from build123d import *

# Parameters (mm, degrees)
BOSS_EXTRUDE1_DEPTH      = 1.27
REVOLVE3_ANGLE           = 90
SKETCH6_W                = 4.862612613
SKETCH6_H                = 1.27
BOSS_EXTRUDE3_DEPTH      = 7.935530078
BOSS_EXTRUDE4_DEPTH      = 3.81
BOSS_EXTRUDE4_DEPTH_BACK = 6.35
SKETCH10_W               = 4.862612613
SKETCH10_H               = 7.935530078
FILLET7_R                = 5.08
FILLET10_R               = 5.08
SKETCH13_R               = 1.651
CUT_EXTRUDE2_DEPTH       = 55.372
SKETCH14_W               = 2.286
SKETCH14_H               = 11.368095807
CUT_EXTRUDE3_DEPTH       = 55.372
FILLET15_RADIUS          = 3.967765039
FILLET15_LENGTH          = 2.576612613
FILLET16_RADIUS          = 3.967765039
FILLET16_LENGTH          = 2.576612613
CUT_EXTRUDE4_DEPTH       = 55.372
CUT_EXTRUDE7_DEPTH       = 55.88
SKETCH19_W               = 2.576612613
SKETCH19_H               = 3.428576371
BOSS_EXTRUDE5_DEPTH      = 3.81
FILLET17_R               = 3.302
FILLET18_R               = 3.302


with BuildPart() as part:
    # Sketch1 → Boss-Extrude1 (new body)
    with BuildSketch(Plane(origin=(0, 0, 0), x_dir=(1, 0, 0), z_dir=(0, 1, 0))):
        with BuildLine():
            Line((-18.44626818, 0), (-13.583655567, 0))
            ThreePointArc((-13.583655567, 0), (5.056359448, 18.640015015), (23.696374463, 0))
            Line((23.696374463, 0), (28.558987076, 0))
            ThreePointArc((28.558987076, 0), (5.056359448, 23.502627628), (-18.44626818, 0))
        make_face()
    extrude(amount=BOSS_EXTRUDE1_DEPTH)

    # Sketch4 → Revolve3 (revolve)
    with BuildSketch(Plane(origin=(0, 1.27, 0), x_dir=(1, 0, 0), z_dir=(0, 1, 0))):
        with BuildLine():
            Line((23.696374463, 0), (28.014374463, 0))
            ThreePointArc((28.014374463, 0), (5.056359448, 22.958015015), (-17.901655567, 0))
            Line((-17.901655567, 0), (-13.583655567, 0))
            ThreePointArc((-13.583655567, 0), (5.056359448, 18.640015015), (23.696374463, 0))
        make_face()
    revolve(axis=Axis((-17.901655567, 1.27, 0), (1, 0, 0)), revolution_arc=REVOLVE3_ANGLE)

    # Sketch6 → Boss-Extrude3 (add)
    with BuildSketch(Plane.XY):
        with Locations((-16.014961873, 0.635)):
            Rectangle(SKETCH6_W, SKETCH6_H)
        with Locations((26.12768077, 0.635)):
            Rectangle(SKETCH6_W, SKETCH6_H)
    extrude(amount=BOSS_EXTRUDE3_DEPTH)

    # Sketch10 → Boss-Extrude4 (add, two sides: drawn at the far end of the back side and taken through both)
    with BuildSketch(Plane(origin=(0, 1.27, 0), x_dir=(1, 0, 0), z_dir=(0, 1, 0)).offset(-BOSS_EXTRUDE4_DEPTH_BACK)):
        with Locations((-16.014961873, -3.967765039)):
            Rectangle(SKETCH10_W, SKETCH10_H)
        with Locations((26.12768077, -3.967765039)):
            Rectangle(SKETCH10_W, SKETCH10_H)
    extrude(amount=BOSS_EXTRUDE4_DEPTH + BOSS_EXTRUDE4_DEPTH_BACK)

    # Fillet7
    fillet7_edges = [part.edges().sort_by_distance(p)[0] for p in [
        (-16.014961873, 5.08, 7.935530078),
    ]]
    fillet(fillet7_edges, radius=FILLET7_R)

    # Fillet10
    fillet10_edges = [part.edges().sort_by_distance(p)[0] for p in [
        (26.127680769, 5.08, 7.935530078),
    ]]
    fillet(fillet10_edges, radius=FILLET10_R)

    # Sketch13 → Cut-Extrude2 (cut)
    with BuildSketch(Plane.ZY.offset(18.44626818)):
        with Locations((3.428576371, 0)):
            Circle(SKETCH13_R)
    extrude(amount=-CUT_EXTRUDE2_DEPTH, mode=Mode.SUBTRACT)

    # Sketch14 → Cut-Extrude3 (cut)
    with BuildSketch(Plane(origin=(0, 5.08, 0), x_dir=(1, 0, 0), z_dir=(0, 1, 0))):
        with Locations((27.415987076, -5.684047904)):
            Rectangle(SKETCH14_W, SKETCH14_H)
        with Locations((-17.30326818, -5.684047904)):
            Rectangle(SKETCH14_W, SKETCH14_H)
    extrude(amount=-CUT_EXTRUDE3_DEPTH, mode=Mode.SUBTRACT)

    # Fillet15: full round fillet: the end face becomes a half cylinder, R = half its width
    fillet15_face = Plane((24.984680769, -5.08, 3.967765039), x_dir=(1, 0, 0), z_dir=(0, -1, 0))  # on the end face: x along it, z out of the body
    fillet15_slab = fillet15_face.offset(-FILLET15_RADIUS / 2) * Box(FILLET15_LENGTH, 2 * FILLET15_RADIUS, FILLET15_RADIUS, mode=Mode.PRIVATE)  # the body's end, R deep
    fillet15_round = Plane((24.984680769, -1.112234961, 3.967765039), x_dir=(0, -1, 0), z_dir=(1, 0, 0)) * Cylinder(FILLET15_RADIUS, FILLET15_LENGTH, mode=Mode.PRIVATE)  # its axis R under the face
    add(fillet15_slab - fillet15_round, mode=Mode.SUBTRACT)

    # Fillet16: full round fillet: the end face becomes a half cylinder, R = half its width
    fillet16_face = Plane((-14.871961873, -5.08, 3.967765039), x_dir=(-1, 0, 0), z_dir=(0, -1, 0))  # on the end face: x along it, z out of the body
    fillet16_slab = fillet16_face.offset(-FILLET16_RADIUS / 2) * Box(FILLET16_LENGTH, 2 * FILLET16_RADIUS, FILLET16_RADIUS, mode=Mode.PRIVATE)  # the body's end, R deep
    fillet16_round = Plane((-14.871961873, -1.112234961, 3.967765039), x_dir=(0, -1, 0), z_dir=(-1, 0, 0)) * Cylinder(FILLET16_RADIUS, FILLET16_LENGTH, mode=Mode.PRIVATE)  # its axis R under the face
    add(fillet16_slab - fillet16_round, mode=Mode.SUBTRACT)

    # Sketch16 → Cut-Extrude4 (cut)
    with BuildSketch(Plane(origin=(26.272987076, 0, 0), x_dir=(0, 0, -1), z_dir=(1, 0, 0))):
        with BuildLine():
            ThreePointArc((0, 0), (-3.716578938, -3.862364093), (-7.935530078, -0.55611748))
            ThreePointArc((-7.935530078, -0.55611748), (-3.630565744, -5.089731167), (0, 0))
        make_face()
    extrude(amount=-CUT_EXTRUDE4_DEPTH, mode=Mode.SUBTRACT)

    # Sketch18 → Cut-Extrude7 (cut)
    with BuildSketch(Plane(origin=(26.272987076, 0, 0), x_dir=(0, 0, -1), z_dir=(1, 0, 0))):
        with BuildLine():
            Line((-3.428576371, 3.428576371), (0, 3.428576371))
            Line((0, 3.428576371), (0, 5.467356317))
            Line((0, 5.467356317), (-9.031573881, 5.467356317))
            Line((-9.031573881, 5.467356317), (-9.031573881, -4.486785293))
            Line((-9.031573881, -4.486785293), (0, -4.486785293))
            Line((0, -4.486785293), (0, 0))
            ThreePointArc((0, 0), (-5.852945973, -2.424369602), (-3.428576371, 3.428576371))
        make_face()
    extrude(amount=-CUT_EXTRUDE7_DEPTH, mode=Mode.SUBTRACT)

    # Sketch19 → Boss-Extrude5 (add)
    with BuildSketch(Plane(origin=(0, 3.428576371, 0), x_dir=(1, 0, 0), z_dir=(0, 1, 0))):
        with Locations((24.98468077, -1.714288186)):
            Rectangle(SKETCH19_W, SKETCH19_H)
        with Locations((-14.871961874, -1.714288186)):
            Rectangle(SKETCH19_W, SKETCH19_H)
    extrude(amount=BOSS_EXTRUDE5_DEPTH)

    # Fillet17
    fillet17_edges = [part.edges().sort_by_distance(p)[0] for p in [
        (24.984680769, 7.238576371, 3.428576371),
    ]]
    fillet(fillet17_edges, radius=FILLET17_R)

    # Fillet18
    fillet18_edges = [part.edges().sort_by_distance(p)[0] for p in [
        (-14.871961873, 7.238576371, 3.428576371),
    ]]
    fillet(fillet18_edges, radius=FILLET18_R)


solid = part.part
CAD build for the part. Positions are in the model's coordinates, mm. A direction names the side the tool comes from. Give positions to 0.01 mm unless a question says otherwise; leave off trailing zeros. Loops run counter-clockwise (first coordinate to the right, second up) from the corner with the lowest first, then second, coordinate; pieces in that order, holes last. Notation, with made-up numbers: M 26,88.5 L 38,88.5 A34 cw 38,119.5 Z; hole C 35.5,34.5 d5. An arc over 180 degrees is marked long. Write each question's results on one line, items separated by ' | '.
Q1. Probe probe 1 along X at (y, z) = (5.5, 3); probe 2 along X at (y, z) = (1, -10); probe 3 along Z at (x, y) = (26, 0.5). List the from-to ranges inside material, lowest first.
Geometry check:
probe 1: x = -16.16 to -13.58, 23.7 to 26.27 | probe 2: x = -16.21 to -10.67, 20.79 to 26.33 | probe 3: z = -10.66 to 1.86, 5 to 6.82
Q2. Which spindle directions (+Z, -Z, +X, -X, +Y, -Y) get a long thin tool onto all of the face, cutting with end or side? Do faces 1 (the face through (7, 0, -19)), 2 (the face through (4.95, 1.27, -23.12)), 3 (the face through (4.646, 0.626, -18.636)), 4 (the face through (23.696, 2, 3)), 5 (the face through (26.273, 2, 3)). Say none if no direction does.
Geometry check:
face 1: -Z, +X, -X, -Y | face 2: -Z, +Y | face 3: +Z, -Y | face 4: +Z, +Y, -Y | face 5: +Z, +X, +Y, -Y
Q3. Band-saw the part on D-D on y = 4.75. Write the cut outline in (x, z).
Geometry check:
outline: M -17.64,0 A22.69 ccw 27.75,0 L 26.27,0 L 26.27,3.33 L 23.7,3.33 L 23.7,0 L 23.37,0 A18.31 cw -13.26,0 L -13.58,0 L -13.58,3.33 L -16.16,3.33 L -16.16,0 Z
Q4. Mould opens along Z. For faces 6 (the face through (24.97, 0.07, 1.78)), 7 (the face through (-14.89, 0.07, 1.78)), 8 (the face through (5.573, 0.626, -23.497)), 9 (the face through (-13.584, 2, 3)) say: pulls with the +Z half, pulls with the -Z half, needs draft (parallel to the pull), parting line crosses it, or undercut.
Geometry check:
face 6: undercut | face 7: undercut | face 8: pulls with the -Z half | face 9: needs draft
Q5. Band-saw the part on A-A on x = 15.5. Write the cut outline in (y, z), and give its area (3 significant figures).
Geometry check:
outline: M 0,-21.05 L 1.27,-21.05 L 1.27,-20.45 A20.45 ccw 21.72,0 L 16.71,0 A15.44 cw 1.27,-15.44 L 0,-15.44 Z | area: 148 mm²
Q6. Flat gauge pins, fed straight in: P1, Ø7, axis at x = 1, z = -16, coming from the +Y side; P2, Ø1.5, axis at x = -12.5, z = -11.5, coming from the -Y side; P3, Ø5.5, axis at y = 1.5, z = 4, coming from the +X side; P4, Ø5.5, axis at y = -0.5, z = 2, coming from the -X side. Where does each tip first touch, or does it go through?
Geometry check:
P1: stops at y = 20.19 | P2: stops at y = 0 | P3: stops at x = 26.27 | P4: stops at x = -18.45
Q7. Band-saw the part on B-B on x = 24.5. Write the cut outline in (y, z).
Geometry check:
outline: M -1.45,0.32 A4 ccw 0,0 L 0,-13.2 L 1.27,-13.2 L 1.27,-12.21 A12.21 ccw 13.48,0 L 7.24,0 L 7.24,0.13 A3.3 ccw 3.94,3.43 L 3.43,3.43 A3.43 ccw long Z; hole C 0,3.43 d3.3
